```python
from build123d import *

# Parameters (mm, degrees)
CHAMFER1_SIZE           = 4
SKETCH2_R               = 3
CUT_EXTRUDE1_DEPTH      = 16
CUT_EXTRUDE1_DEPTH_BACK = 16


with BuildPart() as part:
    # Sketch1 → Revolve1 (revolve)
    with BuildSketch(Plane.XY):
        Polygon((0, 0), (0, -9.5), (90, -9.5), (90, -15), (110, -15), (110, 0), align=None)
    revolve(axis=Axis((0, 0, 0), (1, 0, 0)))

    # Chamfer1
    chamfer1_edges = [part.edges().sort_by_distance(p)[0] for p in [
        (0, 9.5, 0),
        (90, 15, 0),
        (110, 15, 0),
    ]]
    chamfer(chamfer1_edges, length=CHAMFER1_SIZE)

    # Sketch2 → Cut-Extrude1 (cut, two sides)
    with BuildSketch(Plane.XY) as cut_extrude1_sk:
        with Locations((15, 0)):
            Circle(SKETCH2_R)
    extrude(amount=CUT_EXTRUDE1_DEPTH, mode=Mode.SUBTRACT)
    extrude(cut_extrude1_sk.sketch, amount=-CUT_EXTRUDE1_DEPTH_BACK, mode=Mode.SUBTRACT)


solid = part.part
```
Geometry: final body of the model. Coordinates: model frame, mm. A direction names the side the tool comes from. Round coordinates to 2 decimals unless told otherwise and drop trailing zeros. Order: outer loops, then holes, each group sorted by start corner. A loop starts at its lowest first (then second) coordinate and runs counter-clockwise, first axis right, second up. Notation, with made-up numbers: (64, 62.5) -> (80, 62.5) arc R20 ccw to (80, 72.5) -> close; hole circle Ø1 at (47, -22). An arc over 180 degrees is marked (long way). Write each question's results on one line, items separated by ' | '.
Q1. Pin query (flat end, axial travel): pin 1 Ø8 at (y, z) = (-11.5, 0.5) entering from +X; pin 2 Ø1 at (x, z) = (56, -2) entering from +Y; pin 3 Ø5 at (x, z) = (42.5, 9.5) entering from -Y; pin 4 Ø10 at (x, y) = (87.5, 4) entering from -Z. Return the tip coordinate at first contact, or that it passes through.
Response values:
pin 1: x = 110 | pin 2: y = 9.38 | pin 3: y = -6.42 | pin 4: z = -13.06
Q2. Section query A-A (z = 0). Output: boundary loops of the cut face in (x, y).
Response values:
outline: (0, -5.5) -> (4, -9.5) -> (90, -9.5) -> (90, -11) -> (94, -15) -> (106, -15) -> (110, -11) -> (110, 11) -> (106, 15) -> (94, 15) -> (90, 11) -> (90, 9.5) -> (4, 9.5) -> (0, 5.5) -> close; hole circle Ø6 at (15, 0)
Q3. Section query B-B (y = 0). Output: boundary loops of the cut face in (x, z).
Response values:
outline: (0, -5.5) -> (4, -9.5) -> (12, -9.5) -> (12, 9.5) -> (4, 9.5) -> (0, 5.5) -> close; (18, -9.5) -> (90, -9.5) -> (90, -11) -> (94, -15) -> (106, -15) -> (110, -11) -> (110, 11) -> (106, 15) -> (94, 15) -> (90, 11) -> (90, 9.5) -> (18, 9.5) -> close
Q4. Pull-direction query (Y, two-part tool) for faces 1 (the face through (90.25, 2.44, 10.98)), 2 (the face through (0, 0, 0)), 3 (the face through (12, 0, 0)); classes: released by +Y, released by -Y, zero draft, split by the parting line, or undercut.
Response values:
face 1: split by the parting line | face 2: zero draft | face 3: undercut
Q5. Access query for faces 4 (the face through (90, -10, 0)), 5 (the face through (109.806, -10.677, -3.362)). Directions: +Z, -Z, +X, -X, +Y, -Y. A direction counts if a zero-diameter tool reaches every point of the face in a straight line with its end or side. Return the directions, or none.
Response values:
face 4: -X | face 5: +X
Q6. Section query C-C (x = 33). Output: boundary loops of the cut face in (y, z).
Response values:
outline: circle Ø19 at (0, 0)
Q7. Section query D-D (x = 15). Output: boundary loops of the cut face in (y, z).
Response values:
outline: (-3, -9.01) -> (-3, 9.01) arc R9.5 ccw to start; (3, -9.01) arc R9.5 ccw to (3, 9.01) -> close
Q8. Ray query, line 1 along X through (y, z) = (0, 2); line 2 along X through (y, z) = (-6, -7.5); line 3 along Y through (x, z) = (15, 3.5). Return the intervals inside material, ascending.
Response values:
line 1: 0 to 12, 18 to 110 | line 2: 90 to 110 | line 3: -8.83 to -3, 3 to 8.83
